Input: part model. Units: mm. Frame: model coordinates. Face numbers are marked on the shaded views. A direction names the side the tool comes from. Coordinates: 2 decimals unless noted, no trailing zeros. Order: outer loops, then holes, each group sorted by start corner. A loop starts at its lowest first (then second) coordinate and runs counter-clockwise, first axis right, second up. Notation, with made-up numbers: M -0.75,-38.75 L 43.25,-38.75 A10 cw 43.25,-32.75 Z; hole C -11,75 d5. An arc over 180 degrees is marked long. Answer in a Markdown table with one row per item.
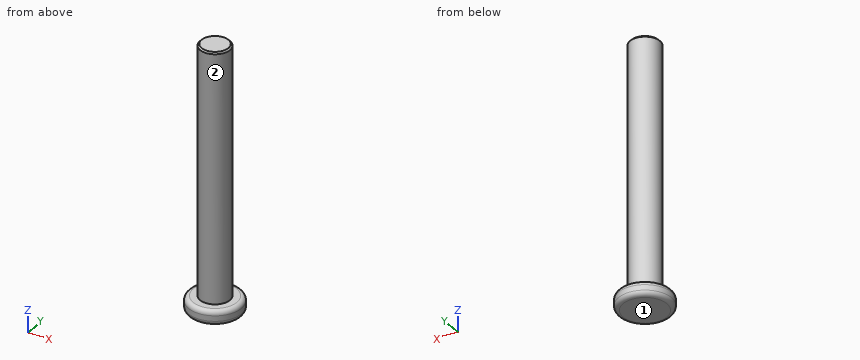
from build123d import *

# Parameters (mm, degrees)
ESQUISSE1_R        = 0.975
BOSS_EXTRU_1_DEPTH = 17.15
ESQUISSE2_R        = 1.725
BOSS_EXTRU_2_DEPTH = 0.95
CONG_1_R           = 0.3
CHANFREIN1_SIZE    = 0.1
SCALE1_SCALE       = 6.5


with BuildPart() as part:
    # Esquisse1 → Boss.-Extru.1 (new body)
    with BuildSketch(Plane.XY):
        Circle(ESQUISSE1_R)
    extrude(amount=BOSS_EXTRU_1_DEPTH)

    # Esquisse2 → Boss.-Extru.2 (add)
    with BuildSketch(Plane(origin=(0, 0, 0), x_dir=(-1, 0, 0), z_dir=(0, 0, -1))):
        Circle(ESQUISSE2_R)
    extrude(amount=-BOSS_EXTRU_2_DEPTH)

    # Congé1
    cong_1_edges = [part.edges().sort_by_distance(p)[0] for p in [
        (1.725, 0, 0),
        (1.725, 0, 0.95),
    ]]
    fillet(cong_1_edges, radius=CONG_1_R)

    # Chanfrein1
    chanfrein1_edges = [part.edges().sort_by_distance(p)[0] for p in [
        (-0.975, 0, 17.15),
    ]]
    chamfer(chanfrein1_edges, length=CHANFREIN1_SIZE)


with BuildPart() as part_1:
    # Scale1: scaled about (0, 0, 7.76650322)
    add(part.part.scale(SCALE1_SCALE).moved(Location((0, 0, -42.71576771))))


solid = part_1.part
1) Material intervals for probe 1 along Z at (x, y) = (-3.5, -7.25); probe 2 along X at (y, z) = (0.5, -12); probe 3 along Y at (x, z) = (0, 52), sorted ascending.
Resolved:
| item | result |
|---|---|
| probe 1 | z = -42.72 to -36.54 |
| probe 2 | x = -6.32 to 6.32 |
| probe 3 | y = -6.34 to 6.34 |
2) Reachability of the marked faces 1 and 2 from +Z, -Z, +X, -X, +Y, -Y: full face, straight path, thin tool, end or side. Return the list, or none.
Resolved:
| item | result |
|---|---|
| face 1 | -Z, +X, -X, +Y, -Y |
| face 2 | +Z |
3) Contact query for flat-ended pins moving along their axis: pin 1 (8 mm diameter, centred on x = -8.5, y = 6.5, fed in from +Z); pin 2 (2 mm diameter, centred on x = -1.5, z = -24.5, fed in from +Y); pin 3 (8 mm diameter, centred on x = 0, z = 15.5, fed in from -Y). Output: stop coordinate, or through.
Resolved:
| item | result |
|---|---|
| pin 1 | stops at z = -36.54 |
| pin 2 | stops at y = 6.32 |
| pin 3 | stops at y = -6.34 |
4) Cut plane C-C, the plane z = -2. Output: boundary loops of the cut face in (x, y) (1 decimal).
Resolved:
| item | result |
|---|---|
| outline | C 0,0 d12.7 |
5) Cut plane A-A, the plane x = 0. Output: boundary loops of the cut face in (y, z).
Resolved:
| item | result |
|---|---|
| outline | M -11.21,-40.77 A1.95 ccw -9.26,-42.72 L 9.26,-42.72 A1.95 ccw 11.21,-40.77 L 11.21,-38.49 A1.95 ccw 9.26,-36.54 L 6.34,-36.54 L 6.34,68.11 L 5.69,68.76 L -5.69,68.76 L -6.34,68.11 L -6.34,-36.54 L -9.26,-36.54 A1.95 ccw -11.21,-38.49 Z |
